from build123d import *

# Parameters (mm, degrees)
ESQUISSE1_W             = 505
ESQUISSE1_H             = 250
ESQUISSE1_R             = 6.5
BOSS_EXTRU_1_DEPTH      = 3
ESQUISSE4_W             = 100
ESQUISSE4_H             = 25
ESQUISSE4_W_2           = 35
ESQUISSE4_H_2           = 84
ESQUISSE4_W_3           = 10
ESQUISSE4_H_3           = 44
ENL_V_MAT_EXTRU_3_DEPTH = 10
CONG_1_R                = 2


with BuildPart() as part:
    # Esquisse1 → Boss.-Extru.1 (new body)
    with BuildSketch(Plane.XY):
        Rectangle(ESQUISSE1_W, ESQUISSE1_H)
        with Locations((131.5, 95)):
            Circle(ESQUISSE1_R, mode=Mode.SUBTRACT)
        with Locations((227.5, 95)):
            Circle(ESQUISSE1_R, mode=Mode.SUBTRACT)
        with Locations((131.5, -105)):
            Circle(ESQUISSE1_R, mode=Mode.SUBTRACT)
        with Locations((227.5, -105)):
            Circle(ESQUISSE1_R, mode=Mode.SUBTRACT)
        with Locations((-128.5, -105)):
            Circle(ESQUISSE1_R, mode=Mode.SUBTRACT)
        with Locations((-128.5, 95)):
            Circle(ESQUISSE1_R, mode=Mode.SUBTRACT)
        with Locations((-224.5, 95)):
            Circle(ESQUISSE1_R, mode=Mode.SUBTRACT)
        with Locations((-224.5, -105)):
            Circle(ESQUISSE1_R, mode=Mode.SUBTRACT)
    extrude(amount=BOSS_EXTRU_1_DEPTH)

    # Esquisse4 → Enlèv. mat.-Extru.3 (cut)
    with BuildSketch(Plane.XY.offset(3)):
        with Locations((-202.5, -30.5)):
            Rectangle(ESQUISSE4_W, ESQUISSE4_H)
        with Locations((-64, -83)):
            Rectangle(ESQUISSE4_W_2, ESQUISSE4_H_2)
        with Locations((247.5, -63)):
            Rectangle(ESQUISSE4_W_3, ESQUISSE4_H_3)
    extrude(amount=-ENL_V_MAT_EXTRU_3_DEPTH, mode=Mode.SUBTRACT)

    # Congé1
    cong_1_edges = [part.edges().sort_by_distance(p)[0] for p in [
        (-152.5, -18, 1.5),
        (-152.5, -43, 1.5),
        (-81.5, -41, 1.5),
        (-46.5, -41, 1.5),
    ]]
    fillet(cong_1_edges, radius=CONG_1_R)


solid = part.part
Geometry check sheet. Reference: the model listing, model coordinates, mm. Give positions to 0.01 mm unless a question says otherwise; leave off trailing zeros. Write each loop counter-clockwise with the first axis right and the second up, starting at its lowest first coordinate (ties: lowest second). Pieces come first, ordered by that corner, then holes. Notation, with made-up numbers: M 75.5,50 L 121.5,50 A19 ccw 121.5,58 Z; hole C 53.5,-18 d4. An arc over 180 degrees is marked long. One line per question, with ' | ' between items.
1. Cross-section at A-A (x = -186). Enter the section's corners in (y, z), plus the area to 3 significant figures.
Ans:
outline: M -125,0 L -43,0 L -43,3 L -125,3 Z; M -18,0 L 125,0 L 125,3 L -18,3 Z | area: 675 mm2
2. Mould release check, pull along X, two halves, no side actions. Record for faces 1 (the face through (126.342, -108.955, 1.479)), 2 (the face through (-133.658, -108.955, 1.479)), 3 (the face through (-4, 2, 3)): released by +X, released by -X, zero draft, split by the parting line, or undercut.
Ans:
face 1: undercut | face 2: undercut | face 3: zero draft
3. Scan lines: line 1 along Y through (x, z) = (227.5, 1.6); line 2 along Y through (x, z) = (-224.5, 1.4); line 3 along X through (y, z) = (-74.5, 0.55). Record each from-to range of solid material in increasing order. Write a range as from..to.
Ans:
line 1: -125..-111.5, -98.5..88.5, 101.5..125 | line 2: -125..-111.5, -98.5..-43, -18..88.5, 101.5..125 | line 3: -252.5..-81.5, -46.5..242.5
4. Cross-section at D-D (y = -105). Enter the section's corners in (x, z), plus the area to 3 significant figures.
Ans:
outline: M -252.5,0 L -231,0 L -231,3 L -252.5,3 Z; M -218,0 L -135,0 L -135,3 L -218,3 Z; M -122,0 L -81.5,0 L -81.5,3 L -122,3 Z; M -46.5,0 L 125,0 L 125,3 L -46.5,3 Z; M 138,0 L 221,0 L 221,3 L 138,3 Z; M 234,0 L 252.5,0 L 252.5,3 L 234,3 Z | area: 1,250 mm2
5. Gauge pin test, flat end, axial feed: pin 1 (0.9 mm diameter, centred on y = -31, z = 1, fed in from -X). Record the tip position at first contact, or that the pin passes through.
Ans:
pin 1: x = -152.5
6. Cross-section at B-B (z = 1.2). Count the separate pieces of the cut face and the enclosed holes in it, plus the area to 3 significant figures.
Ans:
separate pieces: 1 | enclosed holes: 8 | area: 119,000 mm2
7. Cross-section at C-C (x = 131.5). Enter the section's corners in (y, z), plus the area to 3 significant figures.
Ans:
outline: M -125,0 L -111.5,0 L -111.5,3 L -125,3 Z; M -98.5,0 L 88.5,0 L 88.5,3 L -98.5,3 Z; M 101.5,0 L 125,0 L 125,3 L 101.5,3 Z | area: 672 mm2
